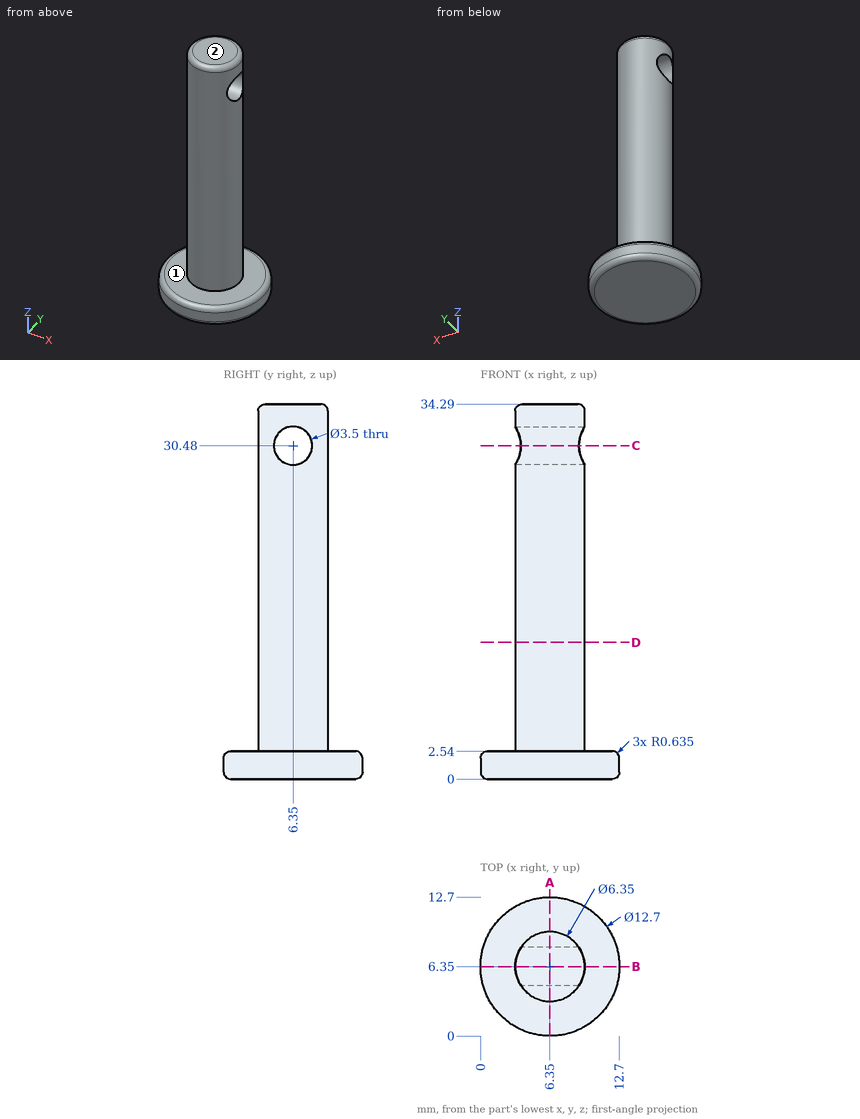
Answer from the drawing. Dimensions are ordinates in mm from the lowest x, y and z of the part. A direction names the side the tool comes from. Round coordinates to 2 decimals unless told otherwise and drop trailing zeros. Loops run counter-clockwise (first coordinate to the right, second up) from the corner with the lowest first, then second, coordinate; pieces in that order, holes last.
Q1. Consider probe 1 along Z at (x, y) = (5, 6.35); probe 2 along Z at (x, y) = (9.25, 3); probe 3 along Y at (x, z) = (5.5, 30.48). Determine where each line is inside the solid, lowest interval first.
Q2. Each of these flat-tipped pins is pushed along its axis until it touches: pin 1 (6 mm diameter, centred on y = 5, z = 16.5, fed in from +X) (3 decimals); pin 2 (5 mm diameter, centred on y = 9, z = 14, fed in from -X); pin 3 (1.5 mm diameter, centred on x = 5.5, z = 17, fed in from +Y). Where does it stop, or does it pass through?
Q3. Which of the six approach directions +Z, -Z, +X, -X, +Y, -Y give full straight-line access (tool end or side, diameter ignored) to the marked faces 1 and 2?
Q4. Section C-C on z = 30.48 is taken. Write down the section's boundary in (x, y) (3 decimals), and give its area (3 significant figures).
Q5. Section D-D on z = 12.5 is taken. Write down the section's boundary in (x, y) (3 decimals), and give its area (3 significant figures).
Q6. Section A-A on x = 6.35 is taken. Write down the section's boundary in (y, z) (3 decimals).
Q7. Section B-B on y = 6.35 is taken. Write down the section's boundary in (x, z) (3 decimals), and give its area (3 significant figures).
Output:
1. probe 1: z = 0 to 28.73, 32.23 to 34.29
1. probe 2: z = 0 to 2.54
1. probe 3: y = 3.29 to 4.6, 8.1 to 9.41
2. pin 1: stops at x = 9.525
2. pin 2: stops at x = 3.18
2. pin 3: stops at y = 9.52
3. face 1: +Z
3. face 2: +Z, +X, -X, +Y, -Y
4. outline: (3.701, 4.6) arc R3.175 ccw to (8.999, 4.6) - close; (3.701, 8.1) - (8.999, 8.1) arc R3.175 ccw to start
4. area: 10.6 mm2
5. outline: circle Ø6.35 at (6.35, 6.35)
5. area: 31.7 mm2
6. outline: (0, 0.635) arc R0.635 ccw to (0.635, 0) - (12.065, 0) arc R0.635 ccw to (12.7, 0.635) - (12.7, 1.905) arc R0.635 ccw to (12.065, 2.54) - (9.525, 2.54) - (9.525, 33.655) arc R0.635 ccw to (8.89, 34.29) - (3.81, 34.29) arc R0.635 ccw to (3.175, 33.655) - (3.175, 2.54) - (0.635, 2.54) arc R0.635 ccw to (0, 1.905) - close; hole circle Ø3.5 at (6.35, 30.48)
7. outline: (0, 0.635) arc R0.635 ccw to (0.635, 0) - (12.065, 0) arc R0.635 ccw to (12.7, 0.635) - (12.7, 1.905) arc R0.635 ccw to (12.065, 2.54) - (9.525, 2.54) - (9.525, 28.73) - (3.175, 28.73) - (3.175, 2.54) - (0.635, 2.54) arc R0.635 ccw to (0, 1.905) - close; (3.175, 32.23) - (9.525, 32.23) - (9.525, 33.655) arc R0.635 ccw to (8.89, 34.29) - (3.81, 34.29) arc R0.635 ccw to (3.175, 33.655) - close
7. area: 211 mm2
